Input: part model. Units: mm. Frame: model coordinates. A direction names the side the tool comes from. Give positions to 0.01 mm unless a question says otherwise; leave off trailing zeros. Order: outer loops, then holes, each group sorted by start corner. A loop starts at its lowest first (then second) coordinate and runs counter-clockwise, first axis right, second up. Notation, with made-up numbers: (24.25, 7) -> (37.25, 7) arc R15 ccw to (37.25, 31) -> close; hole circle Ø2 at (12.25, -25.5). An arc over 180 degrees is marked (long way). Use a Markdown table: item, result. Add a question column.
Autodesk Inventor part; units mm, degrees
ref_plane "YZ Plane" through (0, 0, 0) normal (1, 0, 0) x (0, 1, 0)
ref_plane "XZ Plane" through (0, 0, 0) normal (0, 1, 0) x (-1, 0, 0)
ref_plane "XY Plane" through (0, 0, 0) normal (0, 0, 1) x (1, 0, 0)
sketch "Szkic1" plane through (0, 0, 0) normal (0, 0, 1) x (1, 0, 0)
  line L0 (0, -7.6) -> (0, 45.6)
  line L1 (-8.8, 0) -> (52.8, 0)
  line L2 (0, 0) -> (32, 0)
  line L3 (32, 0) -> (32, 38)
  line L4 (32, 38) -> (0, 38)
  line L5 (0, 38) -> (0, 0)
  circle A0 centre (16, 34) radius 1.5
  line L6 (32, 0) -> (44, 0)
  line L7 (44, 0) -> (44, 22)
  line L8 (44, 22) -> (32, 22)
  line L9 (32, 22) -> (32, 0)
  point P0 (0, 38)
  point P1 (32, 0)
  dimension "d0" = 32
  dimension "d1" = 38
  dimension "d2" = 3
  dimension "d3" = 4
  dimension "d4" = 16
  dimension "d18" = 12
  dimension "d19" = 22
extrude "Wyciągnięcie proste1" add sketch "Szkic1" along normal blind 2
sketch "Szkic2" plane through (0, 0, 2) normal (0, 0, 1) x (1, 0, 0)
  line L0 (0, 38) -> (0, 0)
  line L1 (0, 0) -> (44, 0)
  line L2 (32, 22) -> (32, 38)
  line L3 (32, 38) -> (0, 38)
  circle A0 centre (16, 34) radius 1.5
  line L4 (0, 0) -> (44, 0)
  line L5 (1.5, 0) -> (22.5, 0)
  line L6 (22.5, 0) -> (22.5, 26)
  line L7 (22.5, 26) -> (1.5, 26)
  line L8 (1.5, 26) -> (1.5, 0)
  line L9 (44, 0) -> (44, 22)
  line L10 (44, 22) -> (32, 22)
  point P0 (32, 0)
  dimension "d7" = 26
  dimension "d8" = 21
  dimension "d9" = 1.5
extrude "Wyciągnięcie proste2" add sketch "Szkic2" along normal blind 4 contours L8 L7 L6 L1
sketch "Szkic3" plane through (0, 0, 2) normal (0, 0, 1) x (1, 0, 0)
  line L0 (27.4645, 18.8335) -> (30.4645, 18.8335)
  line L1 (30.4645, 18.8335) -> (30.4645, 0.8335)
  line L2 (30.4645, 0.8335) -> (27.4645, 0.8335)
  line L3 (27.4645, 0.8335) -> (27.4645, 18.8335)
  line L4 (32, 22) -> (32, 38)
  line L5 (21.9813, 36.596) -> (24.8234, 37.5566)
  line L6 (24.8234, 37.5566) -> (30.5867, 20.5042)
  line L7 (30.5867, 20.5042) -> (27.7447, 19.5436)
  line L8 (27.7447, 19.5436) -> (21.9813, 36.596)
  point P0 (0, 0)
  point P1 (32, 0)
  point P2 (26, 22.676)
  point P3 (26, 4.676)
  dimension "d14" = 18
  dimension "d15" = 3
  dimension "d20" = 18
  dimension "d21" = 3
extrude "Wyciągnięcie proste3" add sketch "Szkic3" along normal blind 13
sketch "Szkic4" plane through (30.4645, 0.8335, 2) normal (1, 0, 0) x (0, 0, -1)
  line L0 (0, 18) -> (0, 0)
  line L1 (0, 18) -> (-13, 18)
  line L2 (-13, 0) -> (-13, 18)
  line L3 (0, 0) -> (-13, 0)
  line L4 (-10.5669, 4.9788) -> (-6.5, 4.9788)
  line L5 (-6.5, 4.9788) -> (-6.5, 12.9492)
  line L6 (-6.5, 12.9492) -> (-10.5669, 12.9492)
  line L7 (-10.5669, 12.9492) -> (-10.5669, 4.9788)
  point P0 (2, -0.8335)
extrude "Wyciągnięcie proste4" add sketch "Szkic4" along normal blind 3 contours L7 L6 L5 L4
sketch "Szkic5" plane through (24.8234, 37.5566, 15) normal (0.9473547, 0.320186, 0) x (0, 0, -1)
  line L0 (13, 0) -> (13, -18)
  line L1 (13, 0) -> (0, 0)
  line L2 (0, -18) -> (0, 0)
  line L3 (13, -18) -> (0, -18)
  line L4 (2.5137, -13.1873) -> (6.5, -13.1873)
  line L5 (6.5, -13.1873) -> (6.5, -4.3066)
  line L6 (6.5, -4.3066) -> (2.5137, -4.3066)
  line L7 (2.5137, -4.3066) -> (2.5137, -13.1873)
  point P0 (15, -27.6313)
extrude "Wyciągnięcie proste5" add sketch "Szkic5" along normal blind 3 contours L7 L6 L5 L4
mirror "Odbij2" about plane through (0, 0, 0) normal (0, 1, 0) of "Wyciągnięcie proste1", "Wyciągnięcie proste2", "Wyciągnięcie proste3", "Wyciągnięcie proste4", "Wyciągnięcie proste5"
properties part number "płytka_pcb" material "Tworzywo sztuczne ABS"
Q1. Ray query, line 1 (Y direction, x = 16, z = 0.75); line 2 (Z direction, x = 29.5, y = 26); line 3 (X direction, y = -34, z = 1.25). Return the intervals inside material, ascending.
Q2. Draft query along Z for faces 1 (the flat face through (32, -30, 1)), 2 (the flat face through (32, -10, 8.5)), 3 (the flat face through (32, 10, 12.567)), 4 (the flat face through (22, 1, 0)). Return one class per face: +Z half, -Z half, draft (parallel to the pull), parting line (faces both ways), or undercut.
Q3. Section query A-A (z = 3). Return loops of the section in (x, y).
Q4. Section query C-C (y = 4.5). Return loops of the section in (x, z), plus the area to 3 significant figures.
Q5. Section query D-D (z = 9.25). Give the number of separate pieces and of enclosed holes in the cut face, plus the area to 3 significant figures.
Q6. First-contact query: pin 1 (0.6 mm diameter, centred on y = -30.5, z = 1, fed in from +X); pin 2 (0.9 mm diameter, centred on x = 32, y = 9.5, fed in from +Z); pin 3 (1.2 mm diameter, centred on x = 8.5, z = 3.5, fed in from +Y). Flat tips, straight axial feed; report the tip coordinate or a pass-through.
Q7. Section query B-B (x = 16). Return loops of the section in (y, z).
Q8. Access query for faces 5 (the flat face through (23.422, -37.083, 8.409)), 6 (the flat face through (29, -18.834, 8)), 7 (the flat face through (32, 30, 1)), 8 (the flat face through (38, -22, 1)). Directions: +Z, -Z, +X, -X, +Y, -Y. A direction counts if a zero-diameter tool reaches every point of the face in a straight line with its end or side. Return the directions, or none.
Solution:
| question | item | result |
|---|---|---|
| 1 | line 1 | y = -38 to -35.5, -32.5 to 32.5, 35.5 to 38 |
| 1 | line 2 | z = 0 to 2, 8.5 to 12.49 |
| 1 | line 3 | x = 0 to 14.5, 17.5 to 32 |
| 2 | face 1 | draft |
| 2 | face 2 | undercut |
| 2 | face 3 | +Z half |
| 2 | face 4 | -Z half |
| 3 | outline | (1.5, -26) -> (22.5, -26) -> (22.5, 26) -> (1.5, 26) -> close; (21.98, -36.6) -> (24.82, -37.56) -> (30.59, -20.5) -> (27.74, -19.54) -> close; (21.98, 36.6) -> (27.74, 19.54) -> (30.59, 20.5) -> (24.82, 37.56) -> close; (27.46, -18.83) -> (30.46, -18.83) -> (30.46, -0.83) -> (27.46, -0.83) -> close; (27.46, 0.83) -> (30.46, 0.83) -> (30.46, 18.83) -> (27.46, 18.83) -> close |
| 4 | outline | (0, 0) -> (44, 0) -> (44, 2) -> (30.46, 2) -> (30.46, 15) -> (27.46, 15) -> (27.46, 2) -> (22.5, 2) -> (22.5, 6) -> (1.5, 6) -> (1.5, 2) -> (0, 2) -> close |
| 4 | area | 211 mm² |
| 5 | separate pieces | 4 |
| 5 | enclosed holes | 0 |
| 5 | area | 317 mm² |
| 6 | pin 1 | stops at x = 32 |
| 6 | pin 2 | stops at z = 12.57 |
| 6 | pin 3 | stops at y = 26 |
| 7 | outline | (-38, 0) -> (-35.5, 0) -> (-35.5, 2) -> (-38, 2) -> close; (-32.5, 0) -> (32.5, 0) -> (32.5, 2) -> (26, 2) -> (26, 6) -> (-26, 6) -> (-26, 2) -> (-32.5, 2) -> close; (35.5, 0) -> (38, 0) -> (38, 2) -> (35.5, 2) -> close |
| 8 | face 5 | +Z, -X, -Y |
| 8 | face 6 | +Z, +X |
| 8 | face 7 | +Z, -Z, +X, +Y |
| 8 | face 8 | +Z, -Z, +X, -Y |
